from build123d import *

# Parameters (mm, degrees)
SKETCH_2_W           = 19
SKETCH_2_H           = 19
EXTRUDE_1_DEPTH      = 9.5
FILLET_1_R           = 5
FILLET_2_R           = 5
SKETCH_7_W           = 5.5
SKETCH_7_H           = 4
CUT_EXTRUDE_5_DEPTH  = 1
CUT_EXTRUDE_6_DEPTH  = 1
SKETCH_13_W          = 5.5
SKETCH_13_H          = 4
CUT_EXTRUDE_10_DEPTH = 1
SKETCH_14_W          = 5.5
SKETCH_14_H          = 4
CUT_EXTRUDE_11_DEPTH = 1
SKETCH_15_W          = 5.5
SKETCH_15_H          = 4
CUT_EXTRUDE_12_DEPTH = 1
CUT_EXTRUDE_13_DEPTH = 2
CUT_EXTRUDE_14_DEPTH = 2
CUT_EXTRUDE_START    = 2
CUT_EXTRUDE_15_DEPTH = 2
SKETCH_23_W          = 5.5
SKETCH_23_H          = 4
CUT_EXTRUDE_16_DEPTH = 1
CUT_EXTRUDE_17_DEPTH = 2
SKETCH_27_W          = 10
SKETCH_27_H          = 12
EXTRUDE_2_DEPTH      = 20
SKETCH_28_R          = 4
CUT_EXTRUDE_20_DEPTH = 10


with BuildPart() as part:
    # 草图2 → 凸台-拉伸1 (new, symmetric)
    with BuildSketch(Plane.XY):
        Rectangle(SKETCH_2_W, SKETCH_2_H)
    extrude(amount=EXTRUDE_1_DEPTH, both=True)

    # 圆角1
    fillet_1_edges = [part.edges().sort_by_distance(p)[0] for p in [
        (0, 9.5, 9.5),
    ]]
    fillet(fillet_1_edges, radius=FILLET_1_R)

    # 圆角2
    fillet_2_edges = [part.edges().sort_by_distance(p)[0] for p in [
        (0, -9.5, 9.5),
        (0, -9.5, -9.5),
        (0, 9.5, -9.5),
    ]]
    fillet(fillet_2_edges, radius=FILLET_2_R)

    # 草图7 → 切除-拉伸5 (cut)
    with BuildSketch(Plane(origin=(0, -7.5, 0), x_dir=(-1, 0, 0), z_dir=(0, -1, 0))):
        with Locations((-6.75, 0)):
            Rectangle(SKETCH_7_W, SKETCH_7_H)
        with Locations((6.75, 0)):
            Rectangle(SKETCH_7_W, SKETCH_7_H)
    extrude(amount=CUT_EXTRUDE_5_DEPTH, mode=Mode.SUBTRACT)

    # 草图9 → 切除-拉伸6 (cut)
    with BuildSketch(Plane.XZ.offset(9.5)):
        with BuildLine():
            Line((6, 1), (9.5, 1))
            Line((9.5, 1), (9.5, -1))
            Line((9.5, -1), (6, -1))
            ThreePointArc((6, -1), (5, 0), (6, 1))
        make_face()
        with BuildLine():
            Line((-9.5, 1), (-9.5, -1))
            Line((-9.5, -1), (-6, -1))
            ThreePointArc((-6, -1), (-5, 0), (-6, 1))
            Line((-6, 1), (-9.5, 1))
        make_face()
    extrude(amount=-CUT_EXTRUDE_6_DEPTH, mode=Mode.SUBTRACT)

    # 草图13 → 切除-拉伸10 (cut)
    with BuildSketch(Plane.XY.offset(7.5)):
        with Locations((-6.75, 0)):
            Rectangle(SKETCH_13_W, SKETCH_13_H)
        with Locations((6.75, 0)):
            Rectangle(SKETCH_13_W, SKETCH_13_H)
    extrude(amount=CUT_EXTRUDE_10_DEPTH, mode=Mode.SUBTRACT)

    # 草图14 → 切除-拉伸11 (cut)
    with BuildSketch(Plane(origin=(0, 7.5, 0), x_dir=(1, 0, 0), z_dir=(0, 1, 0))):
        with Locations((-6.75, 0)):
            Rectangle(SKETCH_14_W, SKETCH_14_H)
        with Locations((6.75, 0)):
            Rectangle(SKETCH_14_W, SKETCH_14_H)
    extrude(amount=CUT_EXTRUDE_11_DEPTH, mode=Mode.SUBTRACT)

    # 草图15 → 切除-拉伸12 (cut)
    with BuildSketch(Plane(origin=(0, 0, -7.5), x_dir=(-1, 0, 0), z_dir=(0, 0, -1))):
        with Locations((-6.75, 0)):
            Rectangle(SKETCH_15_W, SKETCH_15_H)
        with Locations((6.75, 0)):
            Rectangle(SKETCH_15_W, SKETCH_15_H)
    extrude(amount=CUT_EXTRUDE_12_DEPTH, mode=Mode.SUBTRACT)

    # 草图20 → 切除-拉伸13 (cut)
    with BuildSketch(Plane(origin=(0, 0, 7.5), x_dir=(-1, 0, 0), z_dir=(0, 0, 1))):
        with BuildLine():
            Line((6, 1), (9.5, 1))
            Line((9.5, 1), (9.5, -1))
            Line((9.5, -1), (6, -1))
            ThreePointArc((6, -1), (5, 0), (6, 1))
        make_face()
        with BuildLine():
            Line((-9.5, 1), (-9.5, -1))
            Line((-9.5, -1), (-6, -1))
            ThreePointArc((-6, -1), (-5, 0), (-6, 1))
            Line((-6, 1), (-9.5, 1))
        make_face()
    extrude(amount=CUT_EXTRUDE_13_DEPTH, mode=Mode.SUBTRACT)

    # 草图21 → 切除-拉伸14 (cut)
    with BuildSketch(Plane(origin=(0, 7.5, 0), x_dir=(-1, 0, 0), z_dir=(0, 1, 0))):
        with BuildLine():
            Line((6, 1), (9.5, 1))
            Line((9.5, 1), (9.5, -1))
            Line((9.5, -1), (6, -1))
            ThreePointArc((6, -1), (5, 0), (6, 1))
        make_face()
        with BuildLine():
            Line((-9.5, 1), (-9.5, -1))
            Line((-9.5, -1), (-6, -1))
            ThreePointArc((-6, -1), (-5, 0), (-6, 1))
            Line((-6, 1), (-9.5, 1))
        make_face()
    extrude(amount=CUT_EXTRUDE_14_DEPTH, mode=Mode.SUBTRACT)

    # 草图22 → 切除-拉伸15 (cut)
    with BuildSketch(Plane(origin=(0, 0, -7.5), x_dir=(1, 0, 0), z_dir=(0, 0, -1)).offset(CUT_EXTRUDE_START)):
        with BuildLine():
            Line((6, 1), (9.5, 1))
            Line((9.5, 1), (9.5, -1))
            Line((9.5, -1), (6, -1))
            ThreePointArc((6, -1), (5, 0), (6, 1))
        make_face()
        with BuildLine():
            Line((-9.5, 1), (-9.5, -1))
            Line((-9.5, -1), (-6, -1))
            ThreePointArc((-6, -1), (-5, 0), (-6, 1))
            Line((-6, 1), (-9.5, 1))
        make_face()
    extrude(amount=-CUT_EXTRUDE_15_DEPTH, mode=Mode.SUBTRACT)

    # 草图23 → 切除-拉伸16 (cut)
    with BuildSketch(Plane(origin=(7.5, 0, 0), x_dir=(0, 0, -1), z_dir=(1, 0, 0))):
        with Locations((-6.75, 0)):
            Rectangle(SKETCH_23_W, SKETCH_23_H)
        with Locations((6.75, 0)):
            Rectangle(SKETCH_23_W, SKETCH_23_H)
    extrude(amount=CUT_EXTRUDE_16_DEPTH, mode=Mode.SUBTRACT)

    # 草图24 → 切除-拉伸17 (cut)
    with BuildSketch(Plane(origin=(7.5, 0, 0), x_dir=(0, 0, 1), z_dir=(1, 0, 0))):
        with BuildLine():
            Line((6, 1), (9.5, 1))
            Line((9.5, 1), (9.5, -1))
            Line((9.5, -1), (6, -1))
            ThreePointArc((6, -1), (5, 0), (6, 1))
        make_face()
        with BuildLine():
            Line((-9.5, 1), (-9.5, -1))
            Line((-9.5, -1), (-6, -1))
            ThreePointArc((-6, -1), (-5, 0), (-6, 1))
            Line((-6, 1), (-9.5, 1))
        make_face()
    extrude(amount=CUT_EXTRUDE_17_DEPTH, mode=Mode.SUBTRACT)

    # 草图27 → 凸台-拉伸2 (add)
    with BuildSketch(Plane.ZY.offset(9.5)):
        Rectangle(SKETCH_27_W, SKETCH_27_H)
    extrude(amount=EXTRUDE_2_DEPTH)

    # 草图28 → 切除-拉伸20 (cut, symmetric)
    with BuildSketch(Plane.XY):
        with Locations(Location((-17.5, 0, 0), (0, 0, 270))):
            Circle(SKETCH_28_R)
    extrude(amount=CUT_EXTRUDE_20_DEPTH, both=True, mode=Mode.SUBTRACT)


solid = part.part
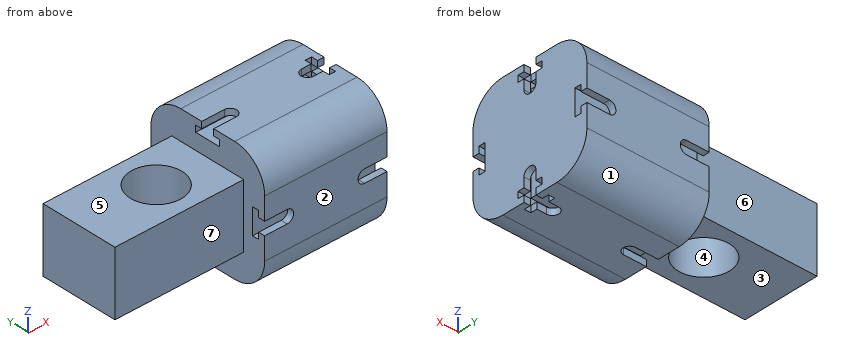
Geometry check sheet. Reference: the model listing, model coordinates, mm. Face numbers are marked on the shaded views. A direction names the side the tool comes from. Give positions to 0.01 mm unless a question says otherwise; leave off trailing zeros. Order: outer loops, then holes, each group sorted by start corner. A loop starts at its lowest first (then second) coordinate and runs counter-clockwise, first axis right, second up.
1) Cross-section at D-D (y = 1.5). Give the number of separate pieces and of enclosed holes in the cut face, then the cut area to 3 significant figures.
Results are:
separate pieces: 4
enclosed holes: 0
area: 456 mm2
2) Cross-section at B-B (z = 0). Record the boundary of the cut face in (x, y).
Results are:
outline: (-29.5, -6) - (-9.5, -6) - (-9.5, -7.5) - (-4, -7.5) - (-4, -8.5) - (-5, -8.5) - (-5, -9.5) - (5, -9.5) - (5, -8.5) - (4, -8.5) - (4, -7.5) - (9.5, -7.5) - (9.5, 7.5) - (4, 7.5) - (4, 8.5) - (5, 8.5) - (5, 9.5) - (-5, 9.5) - (-5, 8.5) - (-4, 8.5) - (-4, 7.5) - (-9.5, 7.5) - (-9.5, 6) - (-29.5, 6) - close; hole circle Ø8 at (-17.5, 0)
3) Draft check along Y on the marked faces 1, 2, 3 and 4. Enter one of: released by +Y, released by -Y, zero draft, split by the parting line, or undercut.
Results are:
face 1: released by +Y
face 2: released by -Y
face 3: zero draft
face 4: undercut
4) Cross-section at A-A (x = -17.5). Record the boundary of the cut face in (y, z).
Results are:
outline: (-6, -5) - (-4, -5) - (-4, 5) - (-6, 5) - close; (4, -5) - (6, -5) - (6, 5) - (4, 5) - close
5) Tool access check on the marked faces 5, 6 and 7. Record the directions out of +Z, -Z, +X, -X, +Y, -Y that give a thin tool (end or side, any length) a straight path to the whole face; none if there is none.
Results are:
face 5: +Z, -X, +Y, -Y
face 6: +Z, -Z, -X, +Y
face 7: +Z, -Z, -X, -Y
6) Cross-section at C-C (x = 2.5). Record the boundary of the cut face in (y, z).
Results are:
outline: (-9.5, -4.5) arc R5 ccw to (-4.5, -9.5) - (4.5, -9.5) arc R5 ccw to (9.5, -4.5) - (9.5, 4.5) arc R5 ccw to (4.5, 9.5) - (-4.5, 9.5) arc R5 ccw to (-9.5, 4.5) - close
7) Material ranges on probe 1 along X at (y, z) = (0, -1); probe 2 along Z at (x, y) = (6, 1.5); probe 3 along Z at (x, y) = (-26.5, 4.5), recorded low to high.
Results are:
probe 1: x = -29.5 to -21.5, -13.5 to 9.5
probe 2: z = -9.5 to -8.5, -7.5 to 7.5, 8.5 to 9.5
probe 3: z = -5 to 5
8) Gauge pin test, flat ends, axial feed: pin 1 (1.1 mm diameter, centred on x = 7, y = -9, fed in from -Z); pin 2 (4 mm diameter, centred on x = -12, y = 1.5, fed in from -Z); pin 3 (0.8 mm diameter, centred on x = 8, y = -1, fed in from +Z). Record the tip position at first contact, or that the pin passes through.
Results are:
pin 1: stops at z = -7.57
pin 2: stops at z = -5
pin 3: stops at z = 4
